from build123d import *

# Parameters (mm, degrees)
F1_DEPTH = 63.5
F2_DEPTH = 25.4
F3_DEPTH = 7.9375
F0_W     = 26.651772843
F0_H     = 19.05
F4_DEPTH = 25.4
F0_H_2   = 4.7498
F5_DEPTH = 25.4
F0_H_3   = 4.7752
F6_DEPTH = 25.4
F7_R     = 6.35


with BuildPart() as f1:
    # F0 (on Front) → F1 (new body, symmetric)
    with BuildSketch(Plane.XZ):
        Polygon((22.225, 9.525), (-41.275, 9.525), (-41.275, -9.525), (41.275, -9.525), (41.275, 9.525), align=None)
    extrude(amount=F1_DEPTH, both=True)

    # F0 (on Front) → F2 (join, symmetric)
    with BuildSketch(Plane.XZ):
        with BuildLine():
            Line((22.225, 27.0002), (22.225, 9.525))
            Line((22.225, 9.525), (41.275, 9.525))
            Line((41.275, 9.525), (41.275, 27.0002))
            ThreePointArc((41.275, 27.0002), (45.9246798487, 38.2255201513), (57.15, 42.8752))
            Line((57.15, 42.8752), (60.325, 42.8752))
            Line((60.325, 42.8752), (60.325, 61.9252))
            Line((60.325, 61.9252), (57.15, 61.9252))
            add(Edge.make_bspline(
                [(49.4302171485, 61.0613300125), (52.1251476125, 61.4486009336), (54.7091322503, 61.7385972485), (57.15, 61.9252)],
                knots=[103.5956862279, 103.5956862279, 103.5956862279, 103.5956862279, 111.5045361635, 111.5045361635, 111.5045361635, 111.5045361635], degree=3))
            ThreePointArc((49.4302171485, 61.0613300125), (29.8610916205, 48.7963259047), (22.225, 27.0002))
        make_face()
    extrude(amount=F2_DEPTH, both=True)

    # F0 (on Front) → F3 (join, symmetric)
    with BuildSketch(Plane.XZ):
        with BuildLine():
            add(Edge.make_bspline(
                [(-41.275, 9.525), (-40.2056240451, 34.2258425008), (14.1301200379, 55.9885827536), (49.4302171485, 61.0613300125)],
                knots=[0, 0, 0, 0, 103.5956862279, 103.5956862279, 103.5956862279, 103.5956862279], degree=3))
            Line((-41.275, 9.525), (22.225, 9.525))
            Line((22.225, 9.525), (22.225, 27.0002))
            ThreePointArc((22.225, 27.0002), (29.8610916205, 48.7963259047), (49.4302171485, 61.0613300125))
        make_face()
    extrude(amount=F3_DEPTH, both=True)

    # F0 (on Front) → F4 (join, symmetric)
    with BuildSketch(Plane.XZ):
        with Locations((73.6508864215, 52.4002)):
            Rectangle(F0_W, F0_H)
    extrude(amount=F4_DEPTH, both=True)

    # F0 (on Front) → F5 (join, symmetric)
    with BuildSketch(Plane.XZ):
        with Locations((73.6508864215, 64.3001)):
            Rectangle(F0_W, F0_H_2)
    extrude(amount=F5_DEPTH, both=True)

    # F0 (on Front) → F6 (join, symmetric)
    with BuildSketch(Plane.XZ):
        with Locations((73.6508864215, 40.4876)):
            Rectangle(F0_W, F0_H_3)
    extrude(amount=F6_DEPTH, both=True)

    # F7
    f7_edges = [f1.edges().sort_by_distance(p)[0] for p in [
        (-41.275, -63.5, 0),
        (41.275, -63.5, 0),
        (41.275, 63.5, 0),
        (-41.275, 63.5, 0),
    ]]
    fillet(f7_edges, radius=F7_R)


solid = f1.part
CAD build for the part. Positions are in the model's coordinates, mm. A direction names the side the tool comes from. Give positions to 0.01 mm unless a question says otherwise; leave off trailing zeros. Write each loop counter-clockwise with the first axis right and the second up, starting at its lowest first coordinate (ties: lowest second). Pieces come first, ordered by that corner, then holes. Notation, with made-up numbers: (74.25, 2) -> (82.25, 2) arc R10 cw to (82.25, 6) -> close; hole circle Ø4 at (65.25, 21.25). An arc over 180 degrees is marked (long way). Return JSON: item names as keys, results as strings.
Item 1: Two-plate mould, pull along X, no slides. Class faces 1 (the flat face through (41.275, -1, 4)), 2 (the flat face through (-1, -1, -9.525)), 3 (the flat face through (60.325, 0, 40)): +X half, -X half, draft (parallel to the pull), parting line (faces both ways), or undercut.
Answer below:
{"face 1": "+X half", "face 2": "draft", "face 3": "undercut"}
Item 2: Drill centre lines: probe 1 along Z at (x, y) = (24, -30.5) (3 decimals); probe 2 along Y at (x, z) = (17, 47.5); probe 3 along X at (y, z) = (-12, 19.5) (3 decimals). Where is each one in solid material? Low to high.
Answer below:
{"probe 1": "z = -9.525 to 9.525", "probe 2": "y = -7.94 to 7.94", "probe 3": "x = 22.225 to 41.275"}
Item 3: Band-saw the part on A-A (z = 5). List the corners of the cut face in (x, y) (3 decimals).
Answer below:
{"outline": "(-41.275, -57.15) arc R6.35 ccw to (-34.925, -63.5) -> (34.925, -63.5) arc R6.35 ccw to (41.275, -57.15) -> (41.275, 57.15) arc R6.35 ccw to (34.925, 63.5) -> (-34.925, 63.5) arc R6.35 ccw to (-41.275, 57.15) -> close"}
Item 4: Band-saw the part on B-B (x = 76). List the corners of the cut face in (y, z) (3 decimals), then the cut area to 3 significant figures.
Answer below:
{"outline": "(-25.4, 38.1) -> (25.4, 38.1) -> (25.4, 66.675) -> (-25.4, 66.675) -> close", "area": "1,450 mm2"}
Item 5: Drop flat-ended pins along their axis: pin 1 (5 mm diameter, centred on y = 1.5, z = 64.5, fed in from -X) (3 decimals); pin 2 (14 mm diameter, centred on y = -15.5, z = 20.5, fed in from -X) (3 decimals); pin 3 (4 mm diameter, centred on y = 25, z = 37, fed in from -X); pin 4 (1.5 mm diameter, centred on x = 52, y = 26.5, fed in from -Z). Give the stop position or say it passes through.
Answer below:
{"pin 1": "stops at x = 60.325", "pin 2": "stops at x = 22.225", "pin 3": "stops at x = 23.15", "pin 4": "passes through"}
Item 6: Tool access for faces 4 (the flat face through (59, 0, 61.925)), 5 (the flat face through (22.225, 17, 18)), 6 (the cylindrical face through (45.8, -0.4, 38.1)), 7 (the flat face through (54, -25.4, 45)): list every direction of +Z, -Z, +X, -X, +Y, -Y with a clear straight run to the whole face (end or side of a thin tool).
Answer below:
{"face 4": "+Z, -X, +Y, -Y", "face 5": "+Z, -X, +Y", "face 6": "-Z, +Y, -Y", "face 7": "+Z, +X, -X, -Y"}
Item 7: Band-saw the part on C-C (y = -48). List the corners of the cut face in (x, z) (3 decimals).
Answer below:
{"outline": "(-41.275, -9.525) -> (41.275, -9.525) -> (41.275, 9.525) -> (-41.275, 9.525) -> close"}
